from build123d import *

# Parameters (mm, degrees)
BOSS_EXTRU_1_DEPTH = 200
TROU_TARAUD_M81_D  = 6.8
D_GAGEMENT_M41_D   = 4.5


with BuildPart() as part:
    # Esquisse1 → Boss.-Extru.1 (new body)
    with BuildSketch(Plane.XY):
        Polygon((0, 0), (0, 84), (45, 84), (45, 79), (5, 79), (5, 0), align=None)
    extrude(amount=BOSS_EXTRU_1_DEPTH)

    # Trou taraudé M81 (through all)
    with Locations(Plane(origin=(0, 79, 0), x_dir=(-1, 0, 0), z_dir=(0, -1, 0))):
        with Locations((-25, -180), (-25, -20)):
            Hole(TROU_TARAUD_M81_D / 2)

    # Dégagement M41 (through all)
    with Locations(Plane.ZY):
        with Locations((175, 5), (100, 5), (25, 5)):
            Hole(D_GAGEMENT_M41_D / 2)


solid = part.part
Verification items for the finished model (mm, model axes). A direction names the side the tool comes from. Give positions to 0.01 mm unless a question says otherwise; leave off trailing zeros. Write each loop counter-clockwise with the first axis right and the second up, starting at its lowest first coordinate (ties: lowest second). Pieces come first, ordered by that corner, then holes.
(1) Cross-section at C-C (x = 24). Enter the section's corners in (y, z), plus the area to 3 significant figures.
(2) Material ranges on line 1 (Z direction, x = 25, y = 80.95); line 2 (X direction, y = 80.35, z = 20); line 3 (Y direction, x = 1, z = 25), recorded low to high.
(3) Gauge pin test, flat ends, axial feed: pin 1 (12 mm diameter, centred on x = 34.5, z = 127, fed in from -Y); pin 2 (6 mm diameter, centred on y = 53.5, z = 96.5, fed in from +X). Record the tip position at first contact, or that the pin passes through.
(4) Cross-section at D-D (z = 153). Enter the section's corners in (x, y), plus the area to 3 significant figures.
(5) Cross-section at B-B (z = 20). Enter the section's corners in (x, y).
(6) Mould release check, pull along Z, two halves, no side actions. Record for faces 3 (the face through (25, 79, 99)), 4 (the face through (4, 58, 0)), 5 (the face through (2.535, 5.676, 22.854)): +Z half, -Z half, draft (parallel to the pull), parting line (faces both ways), or undercut.
(7) Access from +Z, -Z, +X, -X, +Y, -Y to the whole of each face (thin tool, end or side, straight path). Record for faces 1 (the face through (4, 58, 200)), 2 (the face through (5, 40, 99)).
(8) Cross-section at A-A (y = 5). Enter the section's corners in (x, z).
Worked out:
1. outline: (79, 0) - (84, 0) - (84, 16.75) - (79, 16.75) - close; (79, 23.25) - (84, 23.25) - (84, 176.75) - (79, 176.75) - close; (79, 183.25) - (84, 183.25) - (84, 200) - (79, 200) - close
1. area: 935 mm2
2. line 1: z = 0 to 16.6, 23.4 to 176.6, 183.4 to 200
2. line 2: x = 0 to 21.6, 28.4 to 45
2. line 3: y = 0 to 2.75, 7.25 to 84
3. pin 1: stops at y = 79
3. pin 2: stops at x = 5
4. outline: (0, 0) - (5, 0) - (5, 79) - (45, 79) - (45, 84) - (0, 84) - close
4. area: 620 mm2
5. outline: (0, 0) - (5, 0) - (5, 79) - (21.6, 79) - (21.6, 84) - (0, 84) - close; (28.4, 79) - (45, 79) - (45, 84) - (28.4, 84) - close
6. face 3: draft
6. face 4: -Z half
6. face 5: undercut
7. face 1: +Z, +X, -X, +Y, -Y
7. face 2: +Z, -Z, +X, -Y
8. outline: (0, 0) - (5, 0) - (5, 22.75) - (0, 22.75) - close; (0, 27.25) - (5, 27.25) - (5, 97.75) - (0, 97.75) - close; (0, 102.25) - (5, 102.25) - (5, 172.75) - (0, 172.75) - close; (0, 177.25) - (5, 177.25) - (5, 200) - (0, 200) - close
